Autodesk Inventor part; units mm, degrees
ref_plane "YZ Plane" through (0, 0, 0) normal (1, 0, 0) x (0, 1, 0)
ref_plane "XZ Plane" through (0, 0, 0) normal (0, 1, 0) x (-1, 0, 0)
ref_plane "XY Plane" through (0, 0, 0) normal (0, 0, 1) x (1, 0, 0)
sketch "Sketch1" plane through (0, 0, 0) normal (0, 1, 0) x (-1, 0, 0)
  line L0 (0, 17.5) -> (7.366, 17.5)
  line L1 (7.366, 17.5) -> (7.366, -17.5)
  line L2 (7.366, -17.5) -> (0, -17.5)
  line L3 (6.096, 4.754) -> (6.096, -4.754)
  line L4 (0, 4.754) -> (0, 7.802)
  line L5 (6.096, 7.802) -> (6.096, 4.754)
  line L6 (0, -4.754) -> (0, -5.048)
  line L7 (6.096, -7.802) -> (6.096, -4.754)
  line L8 (6.096, 7.802) -> (0, 4.754)
  line L9 (6.096, -7.802) -> (0, -4.754)
  line L10 (0, -17.5) -> (0, -4.754)
  line L11 (0, 4.754) -> (0, 17.5)
  point P0 (0, 0)
  dimension "d0" = 7.366
  dimension "d1" = 35
  dimension "d2" = 17.5
  dimension "d8" = 9.508
  dimension "d9" = 4.754
  dimension "d10" = 3.048
  dimension "d11" = 3.048
  dimension "d12" = 6.096
  dimension "d16" = 15.604
extrude "Shape" add sketch "Sketch1" along normal blind 88.9
sketch "Sketch2" plane through (0, 0, -4.754) normal (1, 0, 0) x (0, 0, -1)
  circle A0 centre (7.5184, 5.08) radius 1.9304
  line L0 (3.048, 0) -> (3.048, 88.9) construction
  line L1 (-12.556, 0) -> (-12.556, 88.9) construction
  line L2 (0, 0) -> (12.746, 0) construction
  line L3 (0, 88.9) -> (12.746, 88.9) construction
  circle A1 centre (7.5184, 31.3267) radius 1.9304
  circle A2 centre (7.5184, 57.5733) radius 1.9304
  circle A3 centre (7.5184, 83.82) radius 1.9304
  circle A4 centre (-17.0264, 5.08) radius 1.9304
  line L4 (-22.254, 0) -> (-9.508, 0) construction
  circle A5 centre (-17.0264, 31.3267) radius 1.9304
  circle A6 centre (-17.0264, 57.5733) radius 1.9304
  circle A7 centre (-17.0264, 83.82) radius 1.9304
  point P0 (-4.754, 0)
  dimension "d19" = 3.8608
  dimension "d20" = 4.4704
  dimension "d21" = 88.9
  dimension "d22" = 5.08
  dimension "d25" = 26.2467
  dimension "d30" = 3.8608
  dimension "d31" = 4.4704
  dimension "d32" = 5.08
  dimension "d35" = 26.2467
extrude "Extrusion2" cut sketch "Sketch2" against normal through all
ref_plane "Work Plane1" through (0, 0, 0) normal (0, 0, -1) x (-1, 0, 0)
equation "\"d11\" = d10"
equation "\"d31\" = d20"
equation "\"d32\" = d22"
properties part number "Coupler receiver"
Can you work these out from the model? Positions are in its coordinate system, mm. A direction names the side the tool comes from. Round coordinates to 2 decimals unless told otherwise and drop trailing zeros. Loops run counter-clockwise (first coordinate to the right, second up) from the corner with the lowest first, then second, coordinate; pieces in that order, holes last. Notation, with made-up numbers: (-22, 79) - (19, 79) arc R13 cw to (19, 94) - close; hole circle Ø3 at (57, -0.5). An arc over 180 degrees is marked (long way). Use CSV: the item, a comma, the result in double quotes. Start each with the question number.
1) If we section it at D-D on z = 12: Write out the boundary of the cut face in (x, y).
2) For faces 1 (the cylindrical face through (-3.631, 85.734, 12.524)), 2 (the flat face through (-6.096, 44, 0)), which set-ups out of +Z, -Z, +X, -X, +Y, -Y let a thin tool reach every point of the face, with its end or its side?
3) If we section it at C-C on y = 39: Write out the boundary of the cut face in (x, z).
4) For pin 1 Ø1 at (y, z) = (18.5, 3.5) entering from +X, with a flat end and sliding along its axis, tell me the tip position at first contact or that it passes through.
5) If we section it at A-A on y = 5.08: Write out the boundary of the cut face in (x, z).
6) Please list where these lines run through material, in increasing order: probe 1 along Y at (x, z) = (-5.75, -11.5); probe 2 along Z at (x, y) = (-4, 83.82); probe 3 along Z at (x, y) = (-3, 85). Write a range as [from, to].
7) If we section it at B-B on x = -5: Count the separate pieces of the cut face and the enclosed holes in it, plus the area to 3 significant figures.
8) We'd pull the mould along Y, two halves only. Please class faces 3 (the flat face through (-7, 0, 0)), 4 (the flat face through (0, 44, -11)), 5 (the cylindrical face through (-3.631, 5.165, -10.344)): released by +Y, released by -Y, zero draft, split by the parting line, or undercut.
Geometry results:
1,outline,"(-7.37, 0) - (0, 0) - (0, 3.17) - (-7.37, 3.17) - close; (-7.37, 6.99) - (0, 6.99) - (0, 29.42) - (-7.37, 29.42) - close; (-7.37, 33.24) - (0, 33.24) - (0, 55.66) - (-7.37, 55.66) - close; (-7.37, 59.48) - (0, 59.48) - (0, 81.91) - (-7.37, 81.91) - close; (-7.37, 85.73) - (0, 85.73) - (0, 88.9) - (-7.37, 88.9) - close"
2,face 1,"+X, -X"
2,face 2,"+Y, -Y"
3,outline,"(-7.37, -17.5) - (0, -17.5) - (0, -4.75) - (-6.1, -7.8) - (-6.1, 7.8) - (0, 4.75) - (0, 17.5) - (-7.37, 17.5) - close"
4,pin 1,"stops at x = -6.1"
5,outline,"(-7.37, -17.5) - (0, -17.5) - (0, -14.2) - (-7.37, -14.2) - close; (-7.37, -10.34) - (0, -10.34) - (0, -4.75) - (-6.1, -7.8) - (-6.1, 7.8) - (0, 4.75) - (0, 10.34) - (-7.37, 10.34) - close; (-7.37, 14.2) - (0, 14.2) - (0, 17.5) - (-7.37, 17.5) - close"
6,probe 1,"y = [0, 3.31], [6.85, 29.56], [33.1, 55.8], [59.34, 82.05], [85.59, 88.9]"
6,probe 2,"z = [-17.5, -14.2], [-10.34, -6.75], [6.75, 10.34], [14.2, 17.5]"
6,probe 3,"z = [-17.5, -13.8], [-10.74, -6.25], [6.25, 10.74], [13.8, 17.5]"
7,separate pieces,"2"
7,enclosed holes,"8"
7,area,"1,730 mm2"
8,face 3,"released by -Y"
8,face 4,"zero draft"
8,face 5,"undercut"
